For this review, take the finished solid that the model builds, in its own axes (mm). A direction names the side the tool comes from. Give positions to 0.01 mm unless a question says otherwise; leave off trailing zeros. Loops run counter-clockwise (first coordinate to the right, second up) from the corner with the lowest first, then second, coordinate; pieces in that order, holes last. Notation, with made-up numbers: (21, 19.5) - (36, 19.5) arc R8 ccw to (36, 23.5) - close; hole circle Ø2 at (78.5, -8.5). An arc over 180 degrees is marked (long way). Answer as CSV lines item,"result".
from build123d import *

# Parameters (mm, degrees)
SKETCH1_R           = 5
BOSS_EXTRUDE1_DEPTH = 220
SKETCH4_R           = 3.2
BOSS_EXTRUDE3_DEPTH = 6
BOSS_EXTRUDE4_DEPTH = 220
SKETCH5_R           = 1.37
CUT_EXTRUDE1_DEPTH  = 7
SKETCH6_R           = 1.37
CUT_EXTRUDE2_DEPTH  = 7
SKETCH7_R           = 3.2
CUT_EXTRUDE3_DEPTH  = 6
CUT_EXTRUDE4_DEPTH  = 10.8
CUT_EXTRUDE5_DEPTH  = 10.8
SKETCH11_R          = 2
CUT_EXTRUDE6_DEPTH  = 7
SKETCH12_R          = 2
CUT_EXTRUDE7_DEPTH  = 7


with BuildPart() as part:
    # Sketch1 → Boss-Extrude1 (new body)
    with BuildSketch(Plane.XY):
        Circle(SKETCH1_R)
        with BuildLine():
            Line((-4, -3), (-7, -8.196152423))
            Line((-7, -8.196152423), (7, -8.196152423))
            Line((7, -8.196152423), (4, -3))
            ThreePointArc((4, -3), (0, 5), (-4, -3))
        make_face()
        with BuildLine():
            Line((28.8, -3), (31.8, -8.196152423))
            Line((31.8, -8.196152423), (17.8, -8.196152423))
            Line((17.8, -8.196152423), (20.8, -3))
            ThreePointArc((20.8, -3), (24.8, 5), (28.8, -3))
        make_face()
    extrude(amount=BOSS_EXTRUDE1_DEPTH)

    # Sketch4 → Boss-Extrude3 (add)
    with BuildSketch(Plane.XZ.offset(8.196152423)):
        with Locations((0, 196.8)):
            Circle(SKETCH4_R)
        with Locations((24.8, 196.8)):
            Circle(SKETCH4_R)
        with Locations((24.8, 172)):
            Circle(SKETCH4_R)
        with Locations((24.8, 147.2)):
            Circle(SKETCH4_R)
        with Locations((24.8, 122.4)):
            Circle(SKETCH4_R)
        with Locations((24.8, 97.6)):
            Circle(SKETCH4_R)
        with Locations((24.8, 72.8)):
            Circle(SKETCH4_R)
        with Locations((24.8, 48)):
            Circle(SKETCH4_R)
        with Locations((24.8, 23.2)):
            Circle(SKETCH4_R)
        with Locations((0, 172)):
            Circle(SKETCH4_R)
        with Locations((0, 147.2)):
            Circle(SKETCH4_R)
        with Locations((0, 122.4)):
            Circle(SKETCH4_R)
        with Locations((0, 97.6)):
            Circle(SKETCH4_R)
        with Locations((0, 72.8)):
            Circle(SKETCH4_R)
        with Locations((0, 48)):
            Circle(SKETCH4_R)
        with Locations((0, 23.2)):
            Circle(SKETCH4_R)
    extrude(amount=BOSS_EXTRUDE3_DEPTH)

    # Sketch3 → Boss-Extrude4 (add)
    with BuildSketch(Plane.XY.offset(220)):
        Polygon((7, -8.196152423), (17.8, -8.196152423), (18.65, -8.196152423), (18.65, -6.723909236), (6.15, -6.723909236), (6.15, -8.196152423), align=None)
    extrude(amount=-BOSS_EXTRUDE4_DEPTH)

    # Sketch5 → Cut-Extrude1 (cut)
    with BuildSketch(Plane(origin=(0, 0, 0), x_dir=(-1, 0, 0), z_dir=(0, 0, -1))):
        Circle(SKETCH5_R)
        with Locations((-24.8, 0)):
            Circle(SKETCH5_R)
    extrude(amount=-CUT_EXTRUDE1_DEPTH, mode=Mode.SUBTRACT)

    # Sketch6 → Cut-Extrude2 (cut)
    with BuildSketch(Plane.XY.offset(220)):
        Circle(SKETCH6_R)
        with Locations((24.8, 0)):
            Circle(SKETCH6_R)
    extrude(amount=-CUT_EXTRUDE2_DEPTH, mode=Mode.SUBTRACT)

    # Sketch7 → Cut-Extrude3 (cut)
    with BuildSketch(Plane.XZ.offset(14.196152423)):
        with Locations((0, 172)):
            Circle(SKETCH7_R)
        with Locations((24.8, 172)):
            Circle(SKETCH7_R)
        with Locations((24.8, 147.2)):
            Circle(SKETCH7_R)
        with Locations((24.8, 122.4)):
            Circle(SKETCH7_R)
        with Locations((24.8, 97.6)):
            Circle(SKETCH7_R)
        with Locations((24.8, 72.8)):
            Circle(SKETCH7_R)
        with Locations((24.8, 48)):
            Circle(SKETCH7_R)
        with Locations((0, 147.2)):
            Circle(SKETCH7_R)
        with Locations((0, 122.4)):
            Circle(SKETCH7_R)
        with Locations((0, 97.6)):
            Circle(SKETCH7_R)
        with Locations((0, 72.8)):
            Circle(SKETCH7_R)
        with Locations((0, 48)):
            Circle(SKETCH7_R)
    extrude(amount=-CUT_EXTRUDE3_DEPTH, mode=Mode.SUBTRACT)

    # Sketch9 → Cut-Extrude4 (cut)
    with BuildSketch(Plane(origin=(0, 0, 0), x_dir=(-1, 0, 0), z_dir=(0, 0, -1))):
        with BuildLine():
            Line((-28.8, -3), (-31.8, -8.196152423))
            Line((-31.8, -8.196152423), (7, -8.196152423))
            Line((7, -8.196152423), (4, -3))
            ThreePointArc((4, -3), (0, 5), (-4, -3))
            Line((-4, -3), (-6.15, -6.723909236))
            Line((-6.15, -6.723909236), (-18.65, -6.723909236))
            Line((-18.65, -6.723909236), (-20.8, -3))
            ThreePointArc((-20.8, -3), (-24.8, 5), (-28.8, -3))
        make_face()
    extrude(amount=-CUT_EXTRUDE4_DEPTH, mode=Mode.SUBTRACT)

    # Sketch10 → Cut-Extrude5 (cut)
    with BuildSketch(Plane.XY.offset(220)):
        with BuildLine():
            Line((20.8, -3), (18.65, -6.723909236))
            Line((18.65, -6.723909236), (6.15, -6.723909236))
            Line((6.15, -6.723909236), (4, -3))
            ThreePointArc((4, -3), (0, 5), (-4, -3))
            Line((-4, -3), (-7, -8.196152423))
            Line((-7, -8.196152423), (31.8, -8.196152423))
            Line((31.8, -8.196152423), (28.8, -3))
            ThreePointArc((28.8, -3), (24.8, 5), (20.8, -3))
        make_face()
    extrude(amount=-CUT_EXTRUDE5_DEPTH, mode=Mode.SUBTRACT)

    # Sketch11 → Cut-Extrude6 (cut)
    with BuildSketch(Plane.XY.offset(209.2)):
        Circle(SKETCH11_R)
        with Locations((24.8, 0)):
            Circle(SKETCH11_R)
    extrude(amount=-CUT_EXTRUDE6_DEPTH, mode=Mode.SUBTRACT)

    # Sketch12 → Cut-Extrude7 (cut)
    with BuildSketch(Plane(origin=(0, 0, 10.8), x_dir=(-1, 0, 0), z_dir=(0, 0, -1))):
        Circle(SKETCH12_R)
        with Locations((-24.8, 0)):
            Circle(SKETCH12_R)
    extrude(amount=-CUT_EXTRUDE7_DEPTH, mode=Mode.SUBTRACT)


solid = part.part
1) Wall thickness on line 1 (Y direction, x = 0, z = 204.75); line 2 (X direction, y = 0, z = 123); line 3 (X direction, y = 1, z = 63.5): over which ranges is each line inside the solid? List them lowest first. Write a range as from..to.
From the geometry:
line 1,"y = -8.2..-2, 2..5"
line 2,"x = -5..5, 19.8..29.8"
line 3,"x = -4.9..4.9, 19.9..29.7"
2) Draft analysis for pull direction Z (two halves, no side actions). For faces 4 (the flat face through (13, -8.196, 109)), 5 (the flat face through (13, -7, 10.8)), 6 (the cylindrical face through (0, -2, 14)), 7 (the cylindrical face through (24.106, -11.154, 193.676)), state which applies: pulls with the +Z half, pulls with the -Z half, needs draft (parallel to the pull), parting line crosses it, or undercut.
From the geometry:
face 4,"undercut"
face 5,"pulls with the -Z half"
face 6,"needs draft"
face 7,"undercut"
3) Machinability: for faces 1 (the cylindrical face through (22.802, 0.088, 205.749)), 2 (the flat face through (0, 0, 17.8)), 3 (the flat face through (30.3, -5.6, 108.6)), which of the approach directions +Z, -Z, +X, -X, +Y, -Y give a long, thin tool a straight path to every point of the face, cutting with its end or side? Answer none if there is none.
From the geometry:
face 1,"+Z"
face 2,"-Z"
face 3,"+Z, -Z, +X"
4) Consider section A-A on y = 0. Write out the cut boundary in (x, z).
From the geometry:
outline,"(-5, 10.8) - (-2, 10.8) - (-2, 17.8) - (2, 17.8) - (2, 10.8) - (5, 10.8) - (5, 209.2) - (2, 209.2) - (2, 202.2) - (-2, 202.2) - (-2, 209.2) - (-5, 209.2) - close; (19.8, 10.8) - (22.8, 10.8) - (22.8, 17.8) - (26.8, 17.8) - (26.8, 10.8) - (29.8, 10.8) - (29.8, 209.2) - (26.8, 209.2) - (26.8, 202.2) - (22.8, 202.2) - (22.8, 209.2) - (19.8, 209.2) - close"
5) Consider section C-C on z = 69. Write out the cut boundary in (x, y), and give its area (3 significant figures).
From the geometry:
outline,"(-7, -8.2) - (31.8, -8.2) - (28.8, -3) arc R5 ccw (long way) to (20.8, -3) - (18.65, -6.72) - (6.15, -6.72) - (4, -3) arc R5 ccw (long way) to (-4, -3) - close"
area,"266 mm^2"
6) Consider section B-B on x = 24.8. Write out the cut boundary in (y, z), and give its area (3 significant figures).
From the geometry:
outline,"(-14.2, 20) - (-8.2, 20) - (-8.2, 10.8) - (-2, 10.8) - (-2, 17.8) - (2, 17.8) - (2, 10.8) - (5, 10.8) - (5, 209.2) - (2, 209.2) - (2, 202.2) - (-2, 202.2) - (-2, 209.2) - (-8.2, 209.2) - (-8.2, 200) - (-14.2, 200) - (-14.2, 193.6) - (-8.2, 193.6) - (-8.2, 26.4) - (-14.2, 26.4) - close"
area,"2,640 mm^2"
7) Insertion check: P1, Ø1.2, axis at x = 0, y = 1, coming from the +Z side; P2, Ø1.2, axis at x = 24, y = -0.5, coming from the -Z side; P3, Ø8, axis at y = 1.5, z = 88.5, coming from the -X side. Each pin has a flat end and moves straight along its axis. Give the tip position at first contact, or say it passes through.
From the geometry:
P1,"stops at z = 202.2"
P2,"stops at z = 17.8"
P3,"stops at x = -5"
8) Consider section D-D on y = -11.75. Write out the cut boundary in (x, z), and give its area (3 significant figures).
From the geometry:
outline,"circle Ø6.4 at (0, 23.2); circle Ø6.4 at (0, 196.8); circle Ø6.4 at (24.8, 23.2); circle Ø6.4 at (24.8, 196.8)"
area,"129 mm^2"
